Model file for the job. Use its own axes, mm. Give positions to 0.01 mm unless a question says otherwise; leave off trailing zeros. Loops run counter-clockwise (first coordinate to the right, second up) from the corner with the lowest first, then second, coordinate; pieces in that order, holes last. Notation, with made-up numbers: M -24,-32 L 20,-32 A22 ccw 20,-10 Z; hole C 84,87.5 d4. An arc over 180 degrees is marked long. Answer in a Markdown table with one row per item.
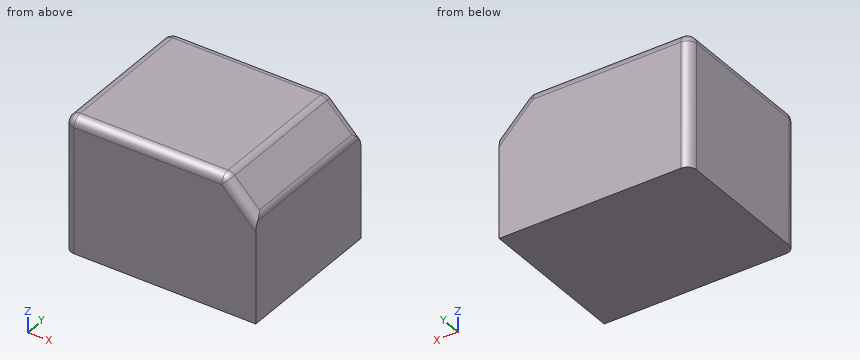
```python
from build123d import *

# Parameters (mm, degrees)
SKETCH049_W     = 20.55
SKETCH049_H     = 16.4
PAD017_DEPTH    = 14.5
SKETCH057_W     = 30
SKETCH057_H     = 20
POCKET032_DEPTH = 16.401
FILLET003_R     = 1


with BuildPart() as part:
    # Sketch049 → Pad017 (new body)
    with BuildSketch(Plane.XY):
        with Locations((-17.425, 38.1)):
            Rectangle(SKETCH049_W, SKETCH049_H)
    extrude(amount=PAD017_DEPTH)

    # Sketch057 (on Face3 of Pad017) → Pocket032 (cut, through all)
    with BuildSketch(Plane.XZ.offset(-29.9)):
        with Locations((-17, 8)):
            Rectangle(SKETCH057_W, SKETCH057_H)
        Polygon((-27.7, 14.5), (-10.4, 14.5), (-7.15, 11.25), (-7.15, 0), (-27.7, 0), align=None, mode=Mode.SUBTRACT)
    extrude(amount=-POCKET032_DEPTH, mode=Mode.SUBTRACT)

    # Fillet003
    fillet003_edges = [part.edges().sort_by_distance(p)[0] for p in [
        (-27.7, 38.1, 14.5),
        (-19.05, 46.3, 14.5),
        (-10.4, 38.1, 14.5),
        (-19.05, 29.9, 14.5),
        (-8.775, 29.9, 12.875),
        (-8.775, 46.3, 12.875),
        (-7.15, 38.1, 11.25),
        (-27.7, 29.9, 7.25),
        (-27.7, 46.3, 7.25),
    ]]
    fillet(fillet003_edges, radius=FILLET003_R)


solid = part.part
```
Q1. Drop a flat-ended pin along its axis: pin 1 (2 mm diameter, centred on x = -21, y = 37, fed in from -Z). Give the stop position or say it passes through.
Reported:
| item | result |
|---|---|
| pin 1 | z = 0 |
Q2. Saw through at A-A (y = 35). Give the cut face in (x, z).
Reported:
| item | result |
|---|---|
| outline | M -27.7,0 L -7.15,0 L -7.15,10.84 A1 ccw -7.44,11.54 L -10.11,14.21 A1 ccw -10.81,14.5 L -26.7,14.5 A1 ccw -27.7,13.5 Z |
Q3. Probe probe 1 along X at (y, z) = (35.25, 13.75); probe 2 along Z at (x, y) = (-26, 30.75); probe 3 along X at (y, z) = (36, 11). List the from-to ranges inside material, lowest first.
Reported:
| item | result |
|---|---|
| probe 1 | -27.67 to -9.65 |
| probe 2 | 0 to 14.49 |
| probe 3 | -27.7 to -7.16 |
